Could you check a few things on this drawing? It's one solid part, dimensions in mm from its lowest x, y, z. A direction names the side the tool comes from. Round coordinates to 2 decimals unless told otherwise and drop trailing zeros. Order: outer loops, then holes, each group sorted by start corner. A loop starts at its lowest first (then second) coordinate and runs counter-clockwise, first axis right, second up. Notation, with made-up numbers: (19, 63) - (35, 63) arc R29 ccw to (35, 92) - close; hole circle Ø11 at (66, 65). An arc over 180 degrees is marked (long way). Use one line per item in the form item = value.
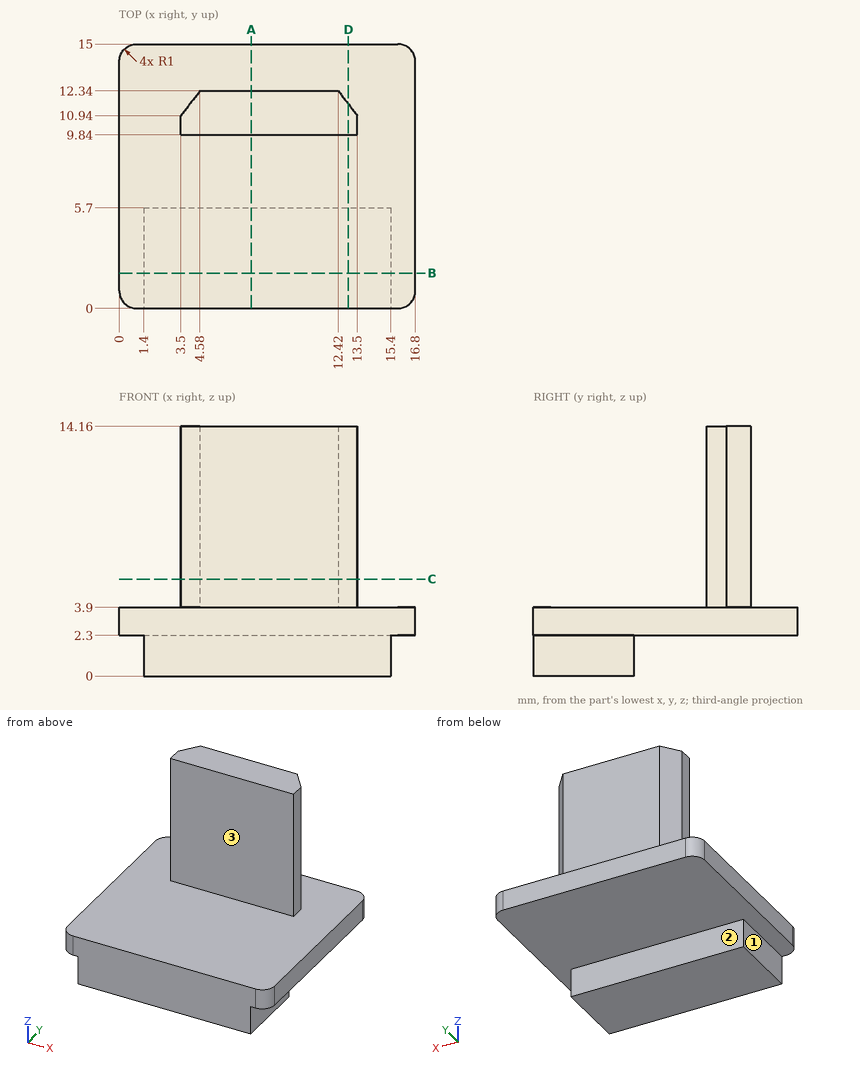
Item 1: For the marked faces 1, 2 and 3, which set-ups out of +Z, -Z, +X, -X, +Y, -Y let a thin tool reach every point of the face, with its end or its side?
Found:
face_1 = -Z, -X, +Y, -Y
face_2 = -Z, +X, -X, +Y
face_3 = +Z, +X, -X, -Y
Item 2: Imagine slicing it at A-A on x = 7.5. Please give me the cut outline in (y, z).
Found:
outline = (0, 0) - (5.7, 0) - (5.7, 2.3) - (15, 2.3) - (15, 3.9) - (12.34, 3.9) - (12.34, 14.16) - (9.84, 14.16) - (9.84, 3.9) - (0, 3.9) - close
Item 3: Imagine slicing it at B-B on y = 2. Please give me the cut outline in (x, z), plus the area to 3 significant figures.
Found:
outline = (0, 2.3) - (1.4, 2.3) - (1.4, 0) - (15.4, 0) - (15.4, 2.3) - (16.8, 2.3) - (16.8, 3.9) - (0, 3.9) - close
area = 59.1 mm2
Item 4: Imagine slicing it at D-D on x = 13. Please give me the cut outline in (y, z), plus the area to 3 significant figures.
Found:
outline = (0, 0) - (5.7, 0) - (5.7, 2.3) - (15, 2.3) - (15, 3.9) - (11.59, 3.9) - (11.59, 14.16) - (9.84, 14.16) - (9.84, 3.9) - (0, 3.9) - close
area = 55.0 mm2
Item 5: Will these pins go through, and if not, where does the flat tip stop? P1, Ø0.9, axis at y = 10.5, z = 7.5, coming from the +X side; P2, Ø7.5, axis at x = 6.5, y = 10.5, coming from the -Z side; P3, Ø0.7, axis at y = 2.5, z = 1, coming from the -X side; P4, Ø1, axis at y = 13, z = 9, coming from the +X side.
Found:
P1 = 13.5
P2 = 2.3
P3 = 1.4
P4 = through
Item 6: I need wall thicknesses on L1, parallel to Z at x = 1.25, y = 5.5; L2, parallel to Z at x = 1.75, y = 1.5; L3, parallel to X at y = 10.5, z = 7.5. Which ranges of each line are inside material? Lowest first, please.
Found:
L1 = 2.3 to 3.9
L2 = 0 to 3.9
L3 = 3.5 to 13.5
Item 7: Imagine slicing it at C-C on z = 5.5. Please give me the cut outline in (x, y), plus the area to 3 significant figures.
Found:
outline = (3.5, 9.84) - (13.5, 9.84) - (13.5, 10.94) - (12.42, 12.34) - (4.58, 12.34) - (3.5, 10.94) - close
area = 23.5 mm2
